```python
from build123d import *

# Parameters (mm, degrees)
CROQUIS1_W              = 78.999998048
CROQUIS1_H              = 74.927002192
SALIENTE_EXTRUIR1_DEPTH = 20.000000019
SALIENTE_EXTRUIR2_DEPTH = 10.311999824
CROQUIS3_W              = 75.000999496
CROQUIS3_H              = 2.000000328
SALIENTE_EXTRUIR3_DEPTH = 8.357999846
CROQUIS4_W              = 24.49000068
CROQUIS4_H              = 6.999999285
CORTAR_EXTRUIR1_DEPTH   = 22.999999881
CROQUIS5_W              = 22.500999272
CROQUIS5_H              = 6.999999285
CORTAR_EXTRUIR2_DEPTH   = 22.999999881
CROQUIS6_W              = 12.001998722
CROQUIS6_H              = 23.004993797
CORTAR_EXTRUIR3_DEPTH   = 21.000000019
CROQUIS7_W              = 24.414002895
CROQUIS7_H              = 6.024999544
SALIENTE_EXTRUIR4_DEPTH = 19.999999553
CROQUIS8_W              = 46.50499858
CROQUIS8_H              = 35.505000502
CORTAR_EXTRUIR4_DEPTH   = 39.669999689
CROQUIS9_W              = 12.004999444
CROQUIS9_H              = 23.004993797
CORTAR_EXTRUIR5_DEPTH   = 21.000000019
CROQUIS10_W             = 15.239998699
CROQUIS10_H             = 15.390999034
CORTAR_EXTRUIR6_DEPTH   = 35.069999285
CROQUIS11_W             = 20.498998463
CROQUIS11_H             = 13.852000004
CORTAR_EXTRUIR7_DEPTH   = 10.311999824
CROQUIS12_W             = 20.499996841
CROQUIS12_H             = 13.852000004
CORTAR_EXTRUIR8_DEPTH   = 10.311999824
CROQUIS13_W             = 5
CROQUIS13_H             = 10
CORTAR_EXTRUIR9_DEPTH   = 2


with BuildPart() as part:
    # Croquis1 → Saliente-Extruir1 (new body)
    with BuildSketch(Plane(origin=(0, 13.269999996, 0), x_dir=(1, 0, 0), z_dir=(0, 1, 0))):
        with Locations((-51.499999128, -37.463501096)):
            Rectangle(CROQUIS1_W, CROQUIS1_H)
    extrude(amount=-SALIENTE_EXTRUIR1_DEPTH)

    # Croquis2 → Saliente-Extruir2 (add)
    with BuildSketch(Plane.XZ.offset(6.730000023)):
        Polygon((-14.878999442, 0), (-88.121004403, 0), (-88.121004403, 19.999999553), (-89.000999928, 19.999999553), (-89.000999928, 21.999999881), (-14.000000432, 21.999999881), (-14.000000432, 19.999999553), (-14.878999442, 19.999999553), align=None)
    extrude(amount=SALIENTE_EXTRUIR2_DEPTH)

    # Croquis3 → Saliente-Extruir3 (add)
    with BuildSketch(Plane.XZ.offset(17.041999847)):
        with Locations((-51.50050018, 20.999999717)):
            Rectangle(CROQUIS3_W, CROQUIS3_H)
    extrude(amount=SALIENTE_EXTRUIR3_DEPTH)

    # Croquis4 → Cortar-Extruir1 (cut, through all)
    with BuildSketch(Plane.XY.offset(21.999999881)):
        with Locations((-26.245000772, -21.900000051)):
            Rectangle(CROQUIS4_W, CROQUIS4_H)
    extrude(amount=-CORTAR_EXTRUIR1_DEPTH, mode=Mode.SUBTRACT)

    # Croquis5 → Cortar-Extruir2 (cut, through all)
    with BuildSketch(Plane.XY.offset(21.999999881)):
        with Locations((-77.750500292, -21.900000051)):
            Rectangle(CROQUIS5_W, CROQUIS5_H)
    extrude(amount=-CORTAR_EXTRUIR2_DEPTH, mode=Mode.SUBTRACT)

    # Croquis6 → Cortar-Extruir3 (cut, through all)
    with BuildSketch(Plane.XZ.offset(6.730000023)):
        with Locations((-84.998998791, 54.500497878)):
            Rectangle(CROQUIS6_W, CROQUIS6_H)
    extrude(amount=-CORTAR_EXTRUIR3_DEPTH, mode=Mode.SUBTRACT)

    # Croquis7 → Saliente-Extruir4 (add)
    with BuildSketch(Plane(origin=(0, 0, 19.999999553), x_dir=(-1, 0, 0), z_dir=(0, 0, -1))):
        with Locations((51.50000006, -20.054499619)):
            Rectangle(CROQUIS7_W, CROQUIS7_H)
    extrude(amount=SALIENTE_EXTRUIR4_DEPTH)

    # Croquis8 → Cortar-Extruir4 (cut, through all)
    with BuildSketch(Plane(origin=(0, 13.269999996, 0), x_dir=(-1, 0, 0), z_dir=(0, 1, 0))):
        with Locations((53.500498645, 43.000498787)):
            Rectangle(CROQUIS8_W, CROQUIS8_H)
    extrude(amount=-CORTAR_EXTRUIR4_DEPTH, mode=Mode.SUBTRACT)

    # Croquis9 → Cortar-Extruir5 (cut, through all)
    with BuildSketch(Plane.XZ.offset(6.730000023)):
        with Locations((-21.000499837, 54.500497878)):
            Rectangle(CROQUIS9_W, CROQUIS9_H)
    extrude(amount=-CORTAR_EXTRUIR5_DEPTH, mode=Mode.SUBTRACT)

    # Croquis10 → Cortar-Extruir6 (cut)
    with BuildSketch(Plane.XZ.offset(23.066999391)):
        with Locations((-51.50000006, 9.319499426)):
            Rectangle(CROQUIS10_W, CROQUIS10_H)
    extrude(amount=-CORTAR_EXTRUIR6_DEPTH, mode=Mode.SUBTRACT)

    # Croquis11 → Cortar-Extruir7 (cut)
    with BuildSketch(Plane.XZ.offset(17.041999847)):
        with Locations((-27.585498988, 9.999999893)):
            Rectangle(CROQUIS11_W, CROQUIS11_H)
    extrude(amount=-CORTAR_EXTRUIR7_DEPTH, mode=Mode.SUBTRACT)

    # Croquis12 → Cortar-Extruir8 (cut)
    with BuildSketch(Plane.XZ.offset(17.041999847)):
        with Locations((-75.486000628, 9.999999893)):
            Rectangle(CROQUIS12_W, CROQUIS12_H)
    extrude(amount=-CORTAR_EXTRUIR8_DEPTH, mode=Mode.SUBTRACT)

    # Croquis13 → Cortar-Extruir9 (cut)
    with BuildSketch(Plane.XY.offset(42.998000979)):
        with Locations((-84.999998152, 8.269999996)):
            Rectangle(CROQUIS13_W, CROQUIS13_H)
    extrude(amount=-CORTAR_EXTRUIR9_DEPTH, mode=Mode.SUBTRACT)


solid = part.part
```
Verification items for the finished model (mm, model axes). A direction names the side the tool comes from. Coordinates: 2 decimals unless noted, no trailing zeros. Loops run counter-clockwise (first coordinate to the right, second up) from the corner with the lowest first, then second, coordinate; pieces in that order, holes last. Notation, with made-up numbers: (87, 42.25) - (143, 42.25) arc R17 cw to (143, 57.25) - close; hole circle Ø5 at (-10, -12.75). An arc over 180 degrees is marked (long way). Answer as a JSON object with one key per item and string values.
(1) Access from +Z, -Z, +X, -X, +Y, -Y to the whole of each face (thin tool, end or side, straight path). Record for faces 1 (the flat face through (-88.121, -12, 10)), 2 (the flat face through (-87.5, 8, 42)), 3 (the flat face through (-26, -18.4, 21)), 4 (the flat face through (-76, -12, 16.926)).
Response:
{"face 1": "-Z, -X, -Y", "face 2": "+Y", "face 3": "+Z, -Z, +X, -Y", "face 4": "-Y"}
(2) Cross-section at C-C, the plane z = 39. Record the boundary of the cut face in (x, y), then the cut area to 3 significant figures.
Response:
{"outline": "(-91, -6.73) - (-76.75, -6.73) - (-76.75, 13.27) - (-91, 13.27) - close; (-30.25, -6.73) - (-12, -6.73) - (-12, 13.27) - (-30.25, 13.27) - close", "area": "650 mm²"}
(3) Go/stop test with flat-tipped pins: pin 1 Ø0.6 at (y, z) = (-13.5, 21) entering from +X; pin 2 Ø3 at (x, y) = (-73.5, -11) entering from +Z; pin 3 Ø6 at (y, z) = (2, 55.5) entering from -X; pin 4 Ø1 at (x, y) = (-36, -20) entering from -Z. Record where each tip stops, or that it passes through.
Response:
{"pin 1": "stops at x = -14", "pin 2": "stops at z = 22", "pin 3": "stops at x = -79", "pin 4": "passes through"}
(4) Mould release check, pull along Z, two halves, no side actions. Record for faces 5 (the flat face through (-52, 3, 74.927)), 6 (the flat face through (-52, -5, 0)), 7 (the flat face through (-66.5, -22, 21)), 8 (the flat face through (-52, -6, 17.015)): pulls with the +Z half, pulls with the -Z half, needs draft (parallel to the pull), parting line crosses it, or undercut.
Response:
{"face 5": "pulls with the +Z half", "face 6": "pulls with the -Z half", "face 7": "needs draft", "face 8": "undercut"}
(5) Scan lines: line 1 along Z through (x, y) = (-47, 10.5) (3 decimals); line 2 along Z through (x, y) = (-54, -8) (3 decimals); line 3 along Z through (x, y) = (-73, -5.5). Record each from-to range of solid material in increasing order.
Response:
{"line 1": "z = 0 to 1.624, 17.015 to 25.248, 60.753 to 74.927", "line 2": "z = 0 to 1.624, 17.015 to 22", "line 3": "z = 0 to 25.25, 60.75 to 74.93"}
(6) Cross-section at B-B, the plane x = -62.5. Record the boundary of the cut face in (y, z), then the cut area to 3 significant figures.
Response:
{"outline": "(-25.4, 20) - (-23.07, 20) - (-23.07, 0) - (13.27, 0) - (13.27, 25.25) - (-6.73, 25.25) - (-6.73, 22) - (-25.4, 22) - close; (-6.73, 60.75) - (13.27, 60.75) - (13.27, 74.93) - (-6.73, 74.93) - close", "area": "1,150 mm²"}
(7) Cross-section at D-D, the plane y = -5. Record the boundary of the cut face in (x, z) (3 decimals), then the cut area to 3 significant figures.
Response:
{"outline": "(-91, 0) - (-12, 0) - (-12, 74.927) - (-91, 74.927) - (-91, 66.003) - (-78.998, 66.003) - (-78.998, 42.998) - (-91, 42.998) - close; hole (-76.753, 25.248) - (-30.248, 25.248) - (-30.248, 60.753) - (-76.753, 60.753) - close; hole (-59.12, 1.624) - (-43.88, 1.624) - (-43.88, 17.015) - (-59.12, 17.015) - close; hole (-27.003, 42.998) - (-14.998, 42.998) - (-14.998, 66.003) - (-27.003, 66.003) - close", "area": "3,480 mm²"}
(8) Cross-section at A-A, the plane z = 47. Record the boundary of the cut face in (x, y), then the cut area to 3 significant figures.
Response:
{"outline": "(-79, -6.73) - (-76.75, -6.73) - (-76.75, 13.27) - (-79, 13.27) - close; (-30.25, -6.73) - (-27, -6.73) - (-27, 13.27) - (-30.25, 13.27) - close; (-15, -6.73) - (-12, -6.73) - (-12, 13.27) - (-15, 13.27) - close", "area": "170 mm²"}
